```python
from build123d import *

# Parameters (mm, degrees)
SKETCH1_W               = 55.14
SKETCH1_H               = 55.14
BOSS_EXTRUDE1_DEPTH     = 17.5
SKETCH2_R               = 3.25
CUT_EXTRUDE1_DEPTH      = 50.8
FILLET1_R               = 5.08
SKETCH3_R               = 3.25
CUT_EXTRUDE2_DEPTH      = 1
CUT_EXTRUDE2_DEPTH_BACK = 18.5
FILLET2_R               = 5.08
SKETCH10_R              = 3.25
CUT_EXTRUDE3_DEPTH      = 1
CUT_EXTRUDE3_DEPTH_BACK = 18.5
SKETCH11_R              = 3.25
CUT_EXTRUDE4_DEPTH      = 1
CUT_EXTRUDE4_DEPTH_BACK = 18.5
FILLET3_R               = 5.08


with BuildPart() as part:
    # Sketch1 → Boss-Extrude1 (new body)
    with BuildSketch(Plane(origin=(0, 0, 0), x_dir=(1, 0, 0), z_dir=(0, 1, 0))):
        Rectangle(SKETCH1_W, SKETCH1_H)
    extrude(amount=BOSS_EXTRUDE1_DEPTH)

    # Sketch2 → Cut-Extrude1 (cut)
    with BuildSketch(Plane(origin=(0, 17.5, 0), x_dir=(1, 0, 0), z_dir=(0, 1, 0))):
        with Locations((-20.82, 20.82)):
            Circle(SKETCH2_R)
    extrude(amount=-CUT_EXTRUDE1_DEPTH, mode=Mode.SUBTRACT)

    # Fillet1
    fillet1_edges = [part.edges().sort_by_distance(p)[0] for p in [
        (-27.57, 8.75, -27.57),
    ]]
    fillet(fillet1_edges, radius=FILLET1_R)

    # Sketch3 → Cut-Extrude2 (cut, two sides)
    with BuildSketch(Plane(origin=(0, 17.5, 0), x_dir=(1, 0, 0), z_dir=(0, 1, 0))) as cut_extrude2_sk:
        with Locations((20.82, 20.82)):
            Circle(SKETCH3_R)
    extrude(amount=CUT_EXTRUDE2_DEPTH, mode=Mode.SUBTRACT)
    extrude(cut_extrude2_sk.sketch, amount=-CUT_EXTRUDE2_DEPTH_BACK, mode=Mode.SUBTRACT)

    # Fillet2
    fillet2_edges = [part.edges().sort_by_distance(p)[0] for p in [
        (27.57, 8.75, -27.57),
    ]]
    fillet(fillet2_edges, radius=FILLET2_R)

    # Sketch10 → Cut-Extrude3 (cut, two sides)
    with BuildSketch(Plane(origin=(0, 17.5, 0), x_dir=(1, 0, 0), z_dir=(0, 1, 0))) as cut_extrude3_sk:
        with Locations((-20.82, -20.82)):
            Circle(SKETCH10_R)
    extrude(amount=CUT_EXTRUDE3_DEPTH, mode=Mode.SUBTRACT)
    extrude(cut_extrude3_sk.sketch, amount=-CUT_EXTRUDE3_DEPTH_BACK, mode=Mode.SUBTRACT)

    # Sketch11 → Cut-Extrude4 (cut, two sides)
    with BuildSketch(Plane(origin=(0, 17.5, 0), x_dir=(1, 0, 0), z_dir=(0, 1, 0))) as cut_extrude4_sk:
        with Locations((20.82, -20.82)):
            Circle(SKETCH11_R)
    extrude(amount=CUT_EXTRUDE4_DEPTH, mode=Mode.SUBTRACT)
    extrude(cut_extrude4_sk.sketch, amount=-CUT_EXTRUDE4_DEPTH_BACK, mode=Mode.SUBTRACT)

    # Fillet3
    fillet3_edges = [part.edges().sort_by_distance(p)[0] for p in [
        (27.57, 8.75, 27.57),
        (-27.57, 8.75, 27.57),
    ]]
    fillet(fillet3_edges, radius=FILLET3_R)


solid = part.part
```
Model file for the job. Use its own axes, mm. Round coordinates to 2 decimals unless told otherwise and drop trailing zeros. Write each loop counter-clockwise with the first axis right and the second up, starting at its lowest first coordinate (ties: lowest second). Pieces come first, ordered by that corner, then holes. Notation, with made-up numbers: M 11.5,47.5 L 29.5,47.5 A25 ccw 29.5,81.5 Z; hole C -19,-39 d8. An arc over 180 degrees is marked long. Put each result on its own line as item: value.
Item 1: Cut at A-A (z = 20.82). List the corners of the cut face in (x, y), and give its area (3 significant figures).
Responses:
outline: M -27.57,0 L -24.07,0 L -24.07,17.5 L -27.57,17.5 Z; M -17.57,0 L 17.57,0 L 17.57,17.5 L -17.57,17.5 Z; M 24.07,0 L 27.57,0 L 27.57,17.5 L 24.07,17.5 Z
area: 737 mm²
Item 2: Mould opens along Z. For faces 1 (the cylindrical face through (-21.243, 8.872, -24.042)), 2 (the flat face through (0, 17.5, 0)), 3 (the cylindrical face through (26.121, 8.872, 26.042)), 4 (the cylindrical face through (-21.5, 8.9, 24)) say: +Z half, -Z half, draft (parallel to the pull), parting line (faces both ways), or undercut.
Responses:
face 1: undercut
face 2: draft
face 3: +Z half
face 4: undercut
Item 3: Cut at C-C (y = 11.5). List the corners of the cut face in (x, z), and give its area (3 significant figures).
Responses:
outline: M -27.57,-22.49 A5.08 ccw -22.49,-27.57 L 22.49,-27.57 A5.08 ccw 27.57,-22.49 L 27.57,22.49 A5.08 ccw 22.49,27.57 L -22.49,27.57 A5.08 ccw -27.57,22.49 Z; hole C -20.82,-20.82 d6.5; hole C -20.82,20.82 d6.5; hole C 20.82,-20.82 d6.5; hole C 20.82,20.82 d6.5
area: 2,890 mm²
Item 4: Probe L1, parallel to X at y = 13, z = -20.82; L2, parallel to Z at x = -22, y = 11.5. List the from-to ranges inside material, lowest first. Write a range as from..to.
Responses:
L1: -27.57..-24.07, -17.57..17.57, 24.07..27.57
L2: -27.57..-23.85, -17.79..17.79, 23.85..27.57
Item 5: Cut at B-B (x = 20.82). List the corners of the cut face in (y, z), and give its area (3 significant figures).
Responses:
outline: M 0,-27.57 L 17.5,-27.57 L 17.5,-24.07 L 0,-24.07 Z; M 0,-17.57 L 17.5,-17.57 L 17.5,17.57 L 0,17.57 Z; M 0,24.07 L 17.5,24.07 L 17.5,27.57 L 0,27.57 Z
area: 737 mm²
